The listing builds one solid part. Answer for the finished solid, in the listing's coordinates (mm). A direction names the side the tool comes from. Coordinates: 2 decimals unless noted, no trailing zeros. Order: outer loops, then holes, each group sorted by start corner. A loop starts at its lowest first (then second) coordinate and runs counter-clockwise, first axis right, second up. Notation, with made-up numbers: (47, 29.5) - (86, 29.5) arc R21 ccw to (86, 49.5) - close; hole circle Ø2 at (-14, -1.5). An arc over 180 degrees is marked (long way). Use one line per item in the form item = value. Start each with the question number.
Item 1: Section A-A, the plane z = 7.5 is taken. Write down the section's boundary in (x, y), and give its area (3 significant figures).
Item 2: Section C-C, the plane y = 6 is taken. Write down the section's boundary in (x, z).
Item 3: A tool of negligible diameter and unlimited length cuts with its end or side. For faces 4 (the cylindrical face through (-1.177, -1.22, 7.395)), 5 (the flat face through (0, 26, 7)), from which of +Z, -Z, +X, -X, +Y, -Y can it reach the whole face along a straight path? Write none if from no direction.
Item 4: Section D-D, the plane z = 12.25 is taken. Write down the section's boundary in (x, y), and give its area (3 significant figures).
Item 5: Each of these flat-tipped pins is pushed along its axis until it touches: pin 1 Ø4 at (y, z) = (42.74, 7.5) entering from -X; pin 2 Ø3 at (x, z) = (10.5, 5) entering from +Y. Where does it stop, or does it pass through?
Item 6: Section B-B, the plane x = 5 is taken. Write down the section's boundary in (y, z).
Item 7: Consider line 1 along Y through (x, z) = (3.5, 2.5); line 2 along X through (y, z) = (-0.75, 7.5). Determine where each line is inside the solid, lowest interval first. Write a range as [from, to].
Item 8: The mould has two halves that part along Y. Classify faces 1 (the flat face through (-1, 50, 7)), 2 (the cylindrical face through (5, -1, 6)), 3 (the cylindrical face through (-0.986, 44.122, 6.925)): released by +Y, released by -Y, zero draft, split by the parting line, or undercut.
from build123d import *

# Parameters (mm, degrees)
SM_BASE_FLANGE_1_DEPTH = 15
SKETCH_6_R             = 1.5
CUT_EXTRUDE_1_DEPTH    = 55.313902456
SKETCH_7_R             = 1.5
CUT_EXTRUDE_2_DEPTH    = 55.313902456


# Sheet-metal steps are written as plain solids
with BuildPart() as part:
    # Sketch 1 → 基体-法兰1 (new body)
    with BuildSketch(Plane.XY):
        with BuildLine():
            Line((0, 50), (0, 0.7366))
            ThreePointArc((0, 0.7366), (0.215745145, 0.215745145), (0.7366, 0))
            Line((0.7366, 0), (15, 0))
            Line((15, 0), (15, -2))
            Line((15, -2), (0.7366, -2))
            ThreePointArc((0.7366, -2), (-1.198468417, -1.198468417), (-2, 0.7366))
            Line((-2, 0.7366), (-2, 50))
            Line((-2, 50), (0, 50))
        make_face()
    extrude(amount=SM_BASE_FLANGE_1_DEPTH)

    # 草图6 → 切除-拉伸1 (cut, through all)
    with BuildSketch(Plane(origin=(0, 0, 0), x_dir=(1, 0, 0), z_dir=(0, 1, 0))):
        with Locations(Location((5, -7.5, 0), (0, 0, 270))):
            Circle(SKETCH_6_R)
    extrude(amount=-CUT_EXTRUDE_1_DEPTH, mode=Mode.SUBTRACT)

    # 草图7 → 切除-拉伸2 (cut, through all)
    with BuildSketch(Plane(origin=(0, 0, 0), x_dir=(0, 0, -1), z_dir=(1, 0, 0))):
        with Locations(Location((-7.5, 42.7366, 0), (0, 0, 90))):
            Circle(SKETCH_7_R)
        with Locations(Location((-7.5, 5.7366, 0), (0, 0, 90))):
            Circle(SKETCH_7_R)
    extrude(amount=-CUT_EXTRUDE_2_DEPTH, mode=Mode.SUBTRACT)


solid = part.part
Response:
q1.outline = (-2, 0.74) arc R2.74 ccw to (0.74, -2) - (3.5, -2) - (3.5, 0) - (0.74, 0) arc R0.74 cw to (0, 0.74) - (0, 4.24) - (-2, 4.24) - close; (-2, 7.24) - (0, 7.24) - (0, 41.24) - (-2, 41.24) - close; (-2, 44.24) - (0, 44.24) - (0, 50) - (-2, 50) - close; (6.5, -2) - (15, -2) - (15, 0) - (6.5, 0) - close
q1.area = 115 mm2
q2.outline = (-2, 0) - (0, 0) - (0, 6.02) - (-2, 6.02) - close; (-2, 8.98) - (0, 8.98) - (0, 15) - (-2, 15) - close
q3.face_4 = +Z, -Z, -X, -Y
q3.face_5 = +Z, -Z, +X, +Y
q4.outline = (-2, 0.74) arc R2.74 ccw to (0.74, -2) - (15, -2) - (15, 0) - (0.74, 0) arc R0.74 cw to (0, 0.74) - (0, 50) - (-2, 50) - close
q4.area = 133 mm2
q5.pin_1 = -2
q5.pin_2 = 0
q6.outline = (-2, 0) - (0, 0) - (0, 6) - (-2, 6) - close; (-2, 9) - (0, 9) - (0, 15) - (-2, 15) - close
q7.line_1 = [-2, 0]
q7.line_2 = [-1.56, 3.5], [6.5, 15]
q8.face_1 = released by +Y
q8.face_2 = zero draft
q8.face_3 = undercut
